Source: CAD feature listing. Evaluate the final solid. Frame: model axes, mm. Face numbers are marked on the shaded views. A direction names the side the tool comes from. Round coordinates to 2 decimals unless told otherwise and drop trailing zeros. Loops run counter-clockwise (first coordinate to the right, second up) from the corner with the lowest first, then second, coordinate; pieces in that order, holes last. Notation, with made-up numbers: M 38,37.25 L 87,37.25 A21 cw 87,58.25 Z; hole C 77,77.5 d5. An arc over 180 degrees is marked long. Answer as a JSON object with one key per item and string values.
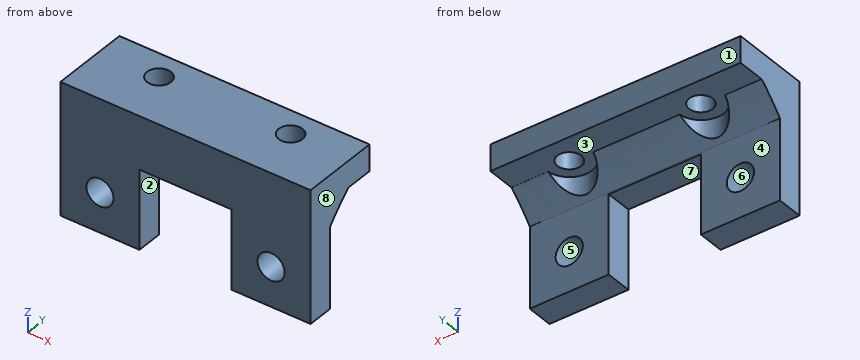
from build123d import *

# Parameters (mm, degrees)
SKETCH1_W           = 30.4
SKETCH1_H           = 6.4
BOSS_EXTRUDE1_DEPTH = 3.2
SKETCH2_W           = 9.6
SKETCH2_H           = 9.6
SKETCH2_R           = 1.65
BOSS_EXTRUDE2_DEPTH = 3.2
SKETCH3_W           = 30.4
SKETCH3_H           = 3.2
BOSS_EXTRUDE3_DEPTH = 6.4
FILLET2_SIZE        = 3
SKETCH4_R           = 1.45
CUT_EXTRUDE1_DEPTH  = 24
SKETCH5_R           = 2.75
CUT_EXTRUDE2_DEPTH  = 4


with BuildPart() as part:
    # Sketch1 → Boss-Extrude1 (new body)
    with BuildSketch(Plane(origin=(0, 0, 0), x_dir=(1, 0, 0), z_dir=(0, 1, 0))):
        with Locations((15.2, -3.2)):
            Rectangle(SKETCH1_W, SKETCH1_H)
    extrude(amount=BOSS_EXTRUDE1_DEPTH)

    # Sketch2 → Boss-Extrude2 (add)
    # profile 1 of 2: a face of its own
    with BuildSketch(Plane(origin=(0, 3.2, 0), x_dir=(1, 0, 0), z_dir=(0, 1, 0))):
        with Locations((4.8, 4.8)):
            Rectangle(SKETCH2_W, SKETCH2_H)
        with Locations(Location((4.8, 4.8, 0), (0, 0, 270))):
            Circle(SKETCH2_R, mode=Mode.SUBTRACT)
    # profile 2 of 2: a face of its own
    with BuildSketch(Plane(origin=(0, 3.2, 0), x_dir=(1, 0, 0), z_dir=(0, 1, 0))):
        with Locations((25.6, 4.8)):
            Rectangle(SKETCH2_W, SKETCH2_H)
        with Locations(Location((25.6, 4.8, 0), (0, 0, 270))):
            Circle(SKETCH2_R, mode=Mode.SUBTRACT)
    extrude(amount=-BOSS_EXTRUDE2_DEPTH)

    # Sketch3 → Boss-Extrude3 (add)
    with BuildSketch(Plane(origin=(0, 3.2, 0), x_dir=(1, 0, 0), z_dir=(0, 1, 0))):
        with Locations((15.2, -4.8)):
            Rectangle(SKETCH3_W, SKETCH3_H)
    extrude(amount=BOSS_EXTRUDE3_DEPTH)

    # Fillet2
    # a fillet whose section is not a circle: 3 mm, written as the material it adds along each edge
    with BuildSketch(Plane(origin=(30.4, 3.2, 3.2), x_dir=(0, 1, 0), z_dir=(-1, 0, 0))) as fillet2_piece_1:
        with BuildLine():
            Bezier((FILLET2_SIZE, 0), (0, 0), (0, FILLET2_SIZE), weights=[1, 0.052631579, 1])
            Line((0, FILLET2_SIZE), (0, 0))
            Line((0, 0), (FILLET2_SIZE, 0))
        make_face()
    extrude(amount=30.4)

    # Sketch4 → Cut-Extrude1 (cut)
    with BuildSketch(Plane.XY.offset(6.4)):
        with Locations((7.2, 6.4)):
            Circle(SKETCH4_R)
        with Locations((23.2, 6.4)):
            Circle(SKETCH4_R)
    extrude(amount=-CUT_EXTRUDE1_DEPTH, mode=Mode.SUBTRACT)

    # Sketch5 → Cut-Extrude2 (cut)
    with BuildSketch(Plane(origin=(0, 0, -0.8), x_dir=(-1, 0, 0), z_dir=(0, 0, -1))):
        with Locations((-23.2, 6.4)):
            Circle(SKETCH5_R)
        with Locations((-7.2, 6.4)):
            Circle(SKETCH5_R)
    extrude(amount=-CUT_EXTRUDE2_DEPTH, mode=Mode.SUBTRACT)


solid = part.part
Item 1: Pull-direction query (Z, two-part tool) for the marked faces 5, 6, 7 and 8; classes: pulls with the +Z half, pulls with the -Z half, needs draft (parallel to the pull), parting line crosses it, or undercut.
Answer sheet:
{"face 5": "undercut", "face 6": "undercut", "face 7": "pulls with the -Z half", "face 8": "needs draft"}
Item 2: Line query: probe 1 along X at (y, z) = (6.25, 5); probe 2 along X at (y, z) = (3, -5); probe 3 along X at (y, z) = (1, -3). Output: solid intervals per line, ascending. Write a range as from..to.
Answer sheet:
{"probe 1": "x = 0..5.76, 8.64..21.76, 24.64..30.4", "probe 2": "x = 0..3.16, 6.44..9.6, 20.8..23.96, 27.24..30.4", "probe 3": "x = 0..9.6, 20.8..30.4"}
Item 3: Section C-C on y = 7.5. Return the cut outline in (x, z), then the cut area to 3 significant figures.
Answer sheet:
{"outline": "M 0,3.2 L 6.26,3.2 L 6.26,6.4 L 0,6.4 Z; M 8.14,3.2 L 22.26,3.2 L 22.26,6.4 L 8.14,6.4 Z; M 24.14,3.2 L 30.4,3.2 L 30.4,6.4 L 24.14,6.4 Z", "area": "85.2 mm²"}
Item 4: Section A-A on z = -7.75. Return the cut outline in (x, y), then the cut area to 3 significant figures.
Answer sheet:
{"outline": "M 0,0 L 9.6,0 L 9.6,3.2 L 0,3.2 Z; M 20.8,0 L 30.4,0 L 30.4,3.2 L 20.8,3.2 Z", "area": "61.4 mm²"}
Item 5: Contact query for flat-ended pins moving along their axis: pin 1 Ø1.7 at (x, y) = (23.2, 6.4) entering from -Z; pin 2 Ø5 at (x, y) = (13.5, 7.5) entering from -Z; pin 3 Ø5.5 at (x, z) = (25.6, -4.8) entering from +Y; pin 4 Ø1.6 at (x, y) = (18, 2) entering from -Z. Output: stop coordinate, or through.
Answer sheet:
{"pin 1": "passes through", "pin 2": "stops at z = 2.15", "pin 3": "stops at y = 3.2", "pin 4": "stops at z = 0"}
Item 6: Section D-D on z = 5.75. Return the cut outline in (x, y).
Answer sheet:
{"outline": "M 0,0 L 30.4,0 L 30.4,9.6 L 0,9.6 Z; hole C 7.2,6.4 d2.9; hole C 23.2,6.4 d2.9"}
Item 7: Section B-B on z = -4.8. Return the cut outline in (x, y).
Answer sheet:
{"outline": "M 0,0 L 3.15,0 L 3.15,3.2 L 0,3.2 Z; M 6.45,0 L 9.6,0 L 9.6,3.2 L 6.45,3.2 Z; M 20.8,0 L 23.95,0 L 23.95,3.2 L 20.8,3.2 Z; M 27.25,0 L 30.4,0 L 30.4,3.2 L 27.25,3.2 Z"}
Item 8: Access query for the marked faces 1, 2, 3 and 4. Directions: +Z, -Z, +X, -X, +Y, -Y. A direction counts if a zero-diameter tool reaches every point of the face in a straight line with its end or side. Return the directions, or none.
Answer sheet:
{"face 1": "+Z, -Z, +X, -X, +Y", "face 2": "-Z, +Y, -Y", "face 3": "-Z, +Y", "face 4": "-Z, +X, -X, +Y"}
